```python
from build123d import *

# Parameters (mm, degrees)
SKETCH1_R           = 12.5
SKETCH1_R_2         = 10.5
BOSS_EXTRUDE1_DEPTH = 10
SKETCH2_R           = 12.5
BOSS_EXTRUDE2_DEPTH = 5
SKETCH3_W           = 2
SKETCH3_H           = 10
BOSS_EXTRUDE3_DEPTH = 15
FILLET1_R           = 5
FILLET2_R           = 5
SKETCH4_R           = 2.5
CUT_EXTRUDE1_DEPTH  = 15


with BuildPart() as part:
    # Sketch1 → Boss-Extrude1 (new body)
    with BuildSketch(Plane(origin=(0, 0, 0), x_dir=(1, 0, 0), z_dir=(0, 1, 0))):
        with Locations(Location((0, 0, 0), (0, 0, 270))):
            Circle(SKETCH1_R)
        with Locations(Location((0, 0, 0), (0, 0, 270))):
            Circle(SKETCH1_R_2, mode=Mode.SUBTRACT)
    extrude(amount=BOSS_EXTRUDE1_DEPTH)

    # Sketch2 → Boss-Extrude2 (add)
    with BuildSketch(Plane(origin=(0, 10, 0), x_dir=(1, 0, 0), z_dir=(0, 1, 0))):
        with Locations(Location((0, 0, 0), (0, 0, 270))):
            Circle(SKETCH2_R)
    extrude(amount=BOSS_EXTRUDE2_DEPTH)

    # Sketch3 → Boss-Extrude3 (add)
    with BuildSketch(Plane(origin=(0, 15, 0), x_dir=(1, 0, 0), z_dir=(0, 1, 0))):
        with Locations((4, 0)):
            Rectangle(SKETCH3_W, SKETCH3_H)
        Rectangle(SKETCH3_W, SKETCH3_H)
        with Locations((-4, 0)):
            Rectangle(SKETCH3_W, SKETCH3_H)
    extrude(amount=BOSS_EXTRUDE3_DEPTH)

    # Fillet1
    fillet1_edges = [part.edges().sort_by_distance(p)[0] for p in [
        (0, 15, -12.5),
    ]]
    fillet(fillet1_edges, radius=FILLET1_R)

    # Fillet2
    fillet2_edges = [part.edges().sort_by_distance(p)[0] for p in [
        (-4, 30, -5),
        (0, 30, -5),
        (4, 30, -5),
        (-4, 30, 5),
        (0, 30, 5),
        (4, 30, 5),
    ]]
    fillet(fillet2_edges, radius=FILLET2_R - 0.0001)  # a hair under: the kernel refuses the full size

    # Sketch4 → Cut-Extrude1 (cut)
    with BuildSketch(Plane(origin=(5, 0, 0), x_dir=(0, 0, -1), z_dir=(1, 0, 0))):
        with Locations((0, 25)):
            Circle(SKETCH4_R)
    extrude(amount=-CUT_EXTRUDE1_DEPTH, mode=Mode.SUBTRACT)


solid = part.part
```
For this review, take the finished solid that the model builds, in its own axes (mm). A direction names the side the tool comes from. Round coordinates to 2 decimals unless told otherwise and drop trailing zeros. Write each loop counter-clockwise with the first axis right and the second up, starting at its lowest first coordinate (ties: lowest second). Pieces come first, ordered by that corner, then holes. Notation, with made-up numbers: (53.5, 11) - (98.5, 11) arc R30 ccw to (98.5, 35) - close; hole circle Ø5 at (61.25, -1). An arc over 180 degrees is marked (long way). Answer as a JSON object with one key per item and string values.
1. Tool access review of faces 1 (the face through (-4, 20, 5)), 2 (the face through (4, 20, -5)), 3 (the face through (3.2, 4.9, 10)), 4 (the face through (3, 21, 0)): name each direction out of +Z, -Z, +X, -X, +Y, -Y from which nothing blocks a thin tool from reaching the whole face with its end or side.
Response values:
{"face 1": "+Z, +X, -X, +Y", "face 2": "-Z, +X, -X, +Y", "face 3": "-Y", "face 4": "+Z, -Z, +Y"}
2. To check wall thickness, follow line 1 along X through (y, z) = (20.75, 2.75); line 2 along Y through (x, z) = (3.8, 0); line 3 along X through (y, z) = (5.5, 0). State the ranges of each line that lie inside material, in increasing order.
Response values:
{"line 1": "x = -5 to -3, -1 to 1, 3 to 5", "line 2": "y = 10 to 22.5, 27.5 to 30", "line 3": "x = -12.5 to -10.5, 10.5 to 12.5"}
3. Draft analysis for pull direction X (two halves, no side actions). For faces 5 (the face through (1, 21, 0)), 6 (the face through (5, 21, 0)), 7 (the face through (0.01, 27.48, 0.33)), state which applies: +X half, -X half, draft (parallel to the pull), parting line (faces both ways), or undercut.
Response values:
{"face 5": "undercut", "face 6": "+X half", "face 7": "draft"}
4. We need section C-C on y = 6.75. Give the boundary of the cut face in (x, z), then the cut area to 3 significant figures.
Response values:
{"outline": "circle Ø25 at (0, 0); hole circle Ø21 at (0, 0)", "area": "145 mm2"}
5. We need section A-A on y = 16.25. Give the boundary of the cut face in (x, z).
Response values:
{"outline": "(-5, -5) - (-3, -5) - (-3, 5) - (-5, 5) - close; (-1, -5) - (1, -5) - (1, 5) - (-1, 5) - close; (3, -5) - (5, -5) - (5, 5) - (3, 5) - close"}
6. For pin 1 Ø8 at (y, z) = (24, 0) entering from +X; pin 2 Ø1.6 at (x, y) = (4, 18.5) entering from -Z; pin 3 Ø2 at (y, z) = (8, 6.5) entering from +X (3 decimals); pin 4 Ø4 at (y, z) = (25, 0) entering from +X, all flat-tipped, find the tip position at first contact; note any pin that passes through.
Response values:
{"pin 1": "stops at x = 5", "pin 2": "stops at z = -5", "pin 3": "stops at x = 11.225", "pin 4": "passes through"}
